```python
from build123d import *

# Parameters (mm, degrees)
SKETCH1_W           = 25
SKETCH1_H           = 15
BOSS_EXTRUDE1_DEPTH = 165
SKETCH2_W           = 19
SKETCH2_H           = 9
CUT_EXTRUDE1_DEPTH  = 263
CUT_EXTRUDE2_DEPTH  = 263
FILLET1_R           = 3


with BuildPart() as part:
    # Sketch1 → Boss-Extrude1 (new body)
    with BuildSketch(Plane.XY):
        Rectangle(SKETCH1_W, SKETCH1_H)
    extrude(amount=BOSS_EXTRUDE1_DEPTH)

    # Sketch2 → Cut-Extrude1 (cut)
    with BuildSketch(Plane.XY.offset(165)):
        Rectangle(SKETCH2_W, SKETCH2_H)
    extrude(amount=-CUT_EXTRUDE1_DEPTH, mode=Mode.SUBTRACT)

    # Sketch3 → Cut-Extrude2 (cut)
    with BuildSketch(Plane(origin=(12.5, 0, 0), x_dir=(0, 0, -1), z_dir=(1, 0, 0))):
        with BuildLine():
            Line((-160, 3.5), (-160, 0.5))
            ThreePointArc((-160, 0.5), (-157.5, -2), (-155, 0.5))
            Line((-155, 0.5), (-155, 3.5))
            Line((-155, 3.5), (-160, 3.5))
        make_face()
        with BuildLine():
            ThreePointArc((-145, 0.5), (-147.5, -2), (-150, 0.5))
            Line((-150, 0.5), (-150, 3.5))
            Line((-150, 3.5), (-145, 3.5))
            Line((-145, 3.5), (-145, 0.5))
        make_face()
        with BuildLine():
            Line((-140, 3.5), (-140, 0.5))
            ThreePointArc((-140, 0.5), (-137.5, -2), (-135, 0.5))
            Line((-135, 0.5), (-135, 3.5))
            Line((-135, 3.5), (-140, 3.5))
        make_face()
        with BuildLine():
            ThreePointArc((-125, 0.5), (-127.5, -2), (-130, 0.5))
            Line((-130, 0.5), (-130, 3.5))
            Line((-130, 3.5), (-125, 3.5))
            Line((-125, 3.5), (-125, 0.5))
        make_face()
        with BuildLine():
            Line((-120, 3.5), (-120, 0.5))
            ThreePointArc((-120, 0.5), (-117.5, -2), (-115, 0.5))
            Line((-115, 0.5), (-115, 3.5))
            Line((-115, 3.5), (-120, 3.5))
        make_face()
        with BuildLine():
            ThreePointArc((-105, 0.5), (-107.5, -2), (-110, 0.5))
            Line((-110, 0.5), (-110, 3.5))
            Line((-110, 3.5), (-105, 3.5))
            Line((-105, 3.5), (-105, 0.5))
        make_face()
        with BuildLine():
            Line((-100, 3.5), (-100, 0.5))
            ThreePointArc((-100, 0.5), (-97.5, -2), (-95, 0.5))
            Line((-95, 0.5), (-95, 3.5))
            Line((-95, 3.5), (-100, 3.5))
        make_face()
        with BuildLine():
            ThreePointArc((-85, 0.5), (-87.5, -2), (-90, 0.5))
            Line((-90, 0.5), (-90, 3.5))
            Line((-90, 3.5), (-85, 3.5))
            Line((-85, 3.5), (-85, 0.5))
        make_face()
        with BuildLine():
            Line((-80, 3.5), (-80, 0.5))
            ThreePointArc((-80, 0.5), (-77.5, -2), (-75, 0.5))
            Line((-75, 0.5), (-75, 3.5))
            Line((-75, 3.5), (-80, 3.5))
        make_face()
        with BuildLine():
            ThreePointArc((-65, 0.5), (-67.5, -2), (-70, 0.5))
            Line((-70, 0.5), (-70, 3.5))
            Line((-70, 3.5), (-65, 3.5))
            Line((-65, 3.5), (-65, 0.5))
        make_face()
        with BuildLine():
            Line((-60, 3.5), (-60, 0.5))
            ThreePointArc((-60, 0.5), (-57.5, -2), (-55, 0.5))
            Line((-55, 0.5), (-55, 3.5))
            Line((-55, 3.5), (-60, 3.5))
        make_face()
        with BuildLine():
            ThreePointArc((-45, 0.5), (-47.5, -2), (-50, 0.5))
            Line((-50, 0.5), (-50, 3.5))
            Line((-50, 3.5), (-45, 3.5))
            Line((-45, 3.5), (-45, 0.5))
        make_face()
        with BuildLine():
            Line((-40, 3.5), (-40, 0.5))
            ThreePointArc((-40, 0.5), (-37.5, -2), (-35, 0.5))
            Line((-35, 0.5), (-35, 3.5))
            Line((-35, 3.5), (-40, 3.5))
        make_face()
        with BuildLine():
            ThreePointArc((-25, 0.5), (-27.5, -2), (-30, 0.5))
            Line((-30, 0.5), (-30, 3.5))
            Line((-30, 3.5), (-25, 3.5))
            Line((-25, 3.5), (-25, 0.5))
        make_face()
        with BuildLine():
            Line((-20, 3.5), (-20, 0.5))
            ThreePointArc((-20, 0.5), (-17.5, -2), (-15, 0.5))
            Line((-15, 0.5), (-15, 3.5))
            Line((-15, 3.5), (-20, 3.5))
        make_face()
        with BuildLine():
            ThreePointArc((-5, 0.5), (-7.5, -2), (-10, 0.5))
            Line((-10, 0.5), (-10, 3.5))
            Line((-10, 3.5), (-5, 3.5))
            Line((-5, 3.5), (-5, 0.5))
        make_face()
        with BuildLine():
            Line((0, 3.5), (0, 0.5))
            ThreePointArc((0, 0.5), (2.5, -2), (5, 0.5))
            Line((5, 0.5), (5, 3.5))
            Line((5, 3.5), (0, 3.5))
        make_face()
        with BuildLine():
            ThreePointArc((15, 0.5), (12.5, -2), (10, 0.5))
            Line((10, 0.5), (10, 3.5))
            Line((10, 3.5), (15, 3.5))
            Line((15, 3.5), (15, 0.5))
        make_face()
        with BuildLine():
            Line((20, 3.5), (20, 0.5))
            ThreePointArc((20, 0.5), (22.5, -2), (25, 0.5))
            Line((25, 0.5), (25, 3.5))
            Line((25, 3.5), (20, 3.5))
        make_face()
        with BuildLine():
            ThreePointArc((35, 0.5), (32.5, -2), (30, 0.5))
            Line((30, 0.5), (30, 3.5))
            Line((30, 3.5), (35, 3.5))
            Line((35, 3.5), (35, 0.5))
        make_face()
        with BuildLine():
            Line((40, 3.5), (40, 0.5))
            ThreePointArc((40, 0.5), (42.5, -2), (45, 0.5))
            Line((45, 0.5), (45, 3.5))
            Line((45, 3.5), (40, 3.5))
        make_face()
        with BuildLine():
            ThreePointArc((55, 0.5), (52.5, -2), (50, 0.5))
            Line((50, 0.5), (50, 3.5))
            Line((50, 3.5), (55, 3.5))
            Line((55, 3.5), (55, 0.5))
        make_face()
    extrude(amount=-CUT_EXTRUDE2_DEPTH, mode=Mode.SUBTRACT)

    # Fillet1
    fillet1_edges = [part.edges().sort_by_distance(p)[0] for p in [
        (12.5, -7.5, 82.5),
        (-12.5, -7.5, 82.5),
        (-12.5, 7.5, 82.5),
        (12.5, 7.5, 82.5),
    ]]
    fillet(fillet1_edges, radius=FILLET1_R)


solid = part.part
```
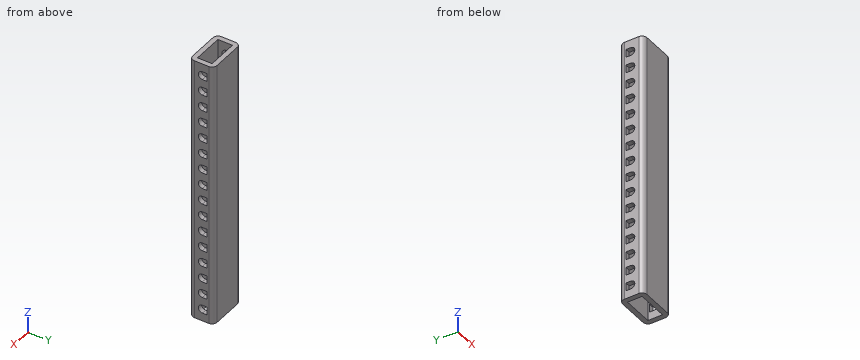
Geometry: final body of the model. Coordinates: model frame, mm. Round coordinates to 2 decimals unless told otherwise and drop trailing zeros. Write each loop counter-clockwise with the first axis right and the second up, starting at its lowest first coordinate (ties: lowest second). Pieces come first, ordered by that corner, then holes.
Item 1: Section query B-B (z = 37.5). Return loops of the section in (x, y), plus the area to 3 significant figures.
Item 2: Material intervals for L1, parallel to Y at x = -3.5, z = 14; L2, parallel to Y at x = 11.5, z = 89.5; L3, parallel to X at y = 5.5, z = 106.5, sorted ascending.
Item 3: Section query C-C (z = 83). Return loops of the section in (x, y).
Item 4: Section query A-A (x = 4.5). Return loops of the section in (y, z).
Item 5: Pin query (flat end, axial travel): P1, Ø0.9, axis at x = -11.5, z = 47, coming from the -Y side; P2, Ø3.5, axis at x = -11.5, z = 77.5, coming from the -Y side; P3, Ø0.9, axis at x = -11, z = 37, coming from the -Y side. Return the tip coordinate at first contact, or that it passes through.
Item 6: Section query D-D (z = 57). Return loops of the section in (x, y).
Completed:
1. outline: (-12.5, -4.5) arc R3 ccw to (-9.5, -7.5) - (9.5, -7.5) arc R3 ccw to (12.5, -4.5) - (12.5, -2) - (9.5, -2) - (9.5, -4.5) - (-9.5, -4.5) - (-9.5, -2) - (-12.5, -2) - close; (-12.5, 3.5) - (-9.5, 3.5) - (-9.5, 4.5) - (9.5, 4.5) - (9.5, 3.5) - (12.5, 3.5) - (12.5, 4.5) arc R3 ccw to (9.5, 7.5) - (-9.5, 7.5) arc R3 ccw to (-12.5, 4.5) - close
1. area: 163 mm2
2. L1: y = -7.5 to -4.5, 4.5 to 7.5
2. L2: y = -6.74 to -1, 3.5 to 6.74
2. L3: x = -12.33 to 12.33
3. outline: (-12.5, -4.5) arc R3 ccw to (-9.5, -7.5) - (9.5, -7.5) arc R3 ccw to (12.5, -4.5) - (12.5, 4.5) arc R3 ccw to (9.5, 7.5) - (-9.5, 7.5) arc R3 ccw to (-12.5, 4.5) - close; hole (-9.5, -4.5) - (9.5, -4.5) - (9.5, 4.5) - (-9.5, 4.5) - close
4. outline: (-7.5, 0) - (-4.5, 0) - (-4.5, 165) - (-7.5, 165) - close; (4.5, 0) - (7.5, 0) - (7.5, 165) - (4.5, 165) - close
5. P1: stops at y = -7.07
5. P2: stops at y = -7.49
5. P3: stops at y = -7.31
6. outline: (-12.5, -4.5) arc R3 ccw to (-9.5, -7.5) - (9.5, -7.5) arc R3 ccw to (12.5, -4.5) - (12.5, -1.95) - (9.5, -1.95) - (9.5, -4.5) - (-9.5, -4.5) - (-9.5, -1.95) - (-12.5, -1.95) - close; (-12.5, 3.5) - (-9.5, 3.5) - (-9.5, 4.5) - (9.5, 4.5) - (9.5, 3.5) - (12.5, 3.5) - (12.5, 4.5) arc R3 ccw to (9.5, 7.5) - (-9.5, 7.5) arc R3 ccw to (-12.5, 4.5) - close
